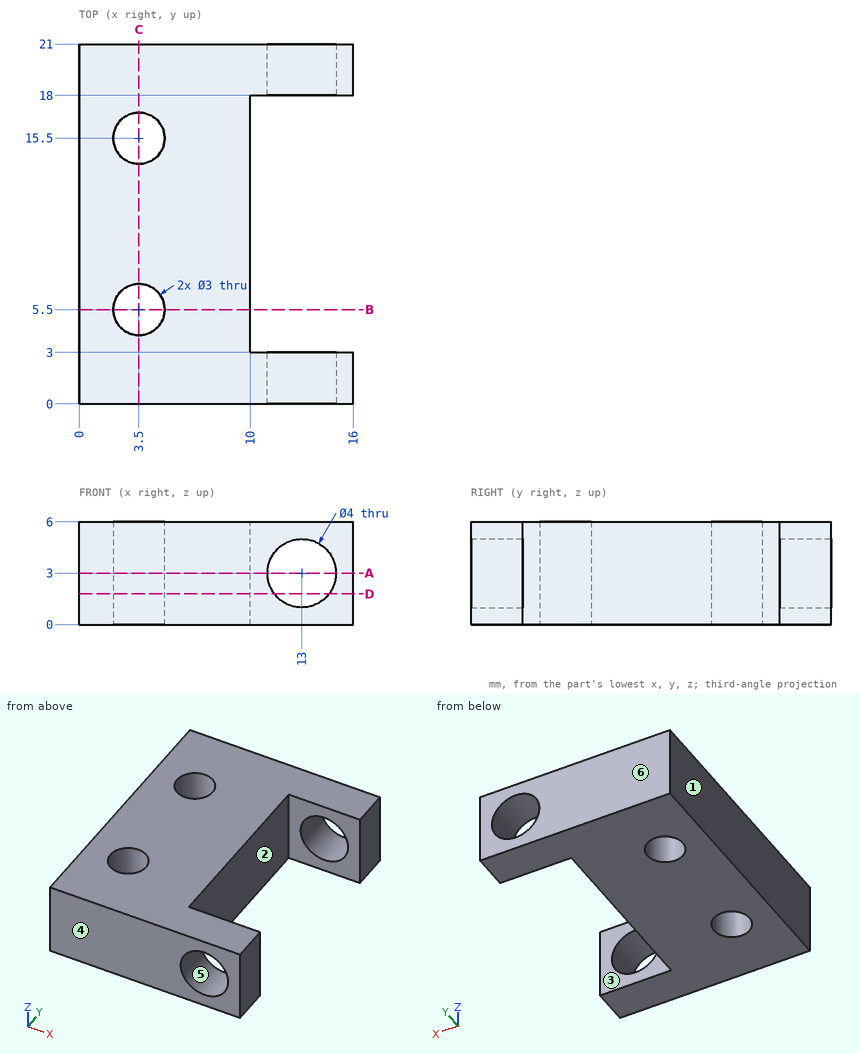
For this review, use the dimensioned drawing (mm, ordinates from the lowest corner) and the shaded views. A direction names the side the tool comes from. Round coordinates to 2 decimals unless told otherwise and drop trailing zeros. Write each loop counter-clockwise with the first axis right and the second up, starting at its lowest first coordinate (ties: lowest second). Pieces come first, ordered by that corner, then holes. Notation, with made-up numbers: M -39.5,-38.5 L 0.5,-38.5 A31 cw 0.5,-3.5 Z; hole C -33.5,4.5 d1. An arc over 180 degrees is marked long. Answer as CSV lines item,"result". Start each with the question number.
Q1. The part is to be moulded in two halves that separate along Y. For the marked faces 3, 4, 5 and 6, say which applies: +Y half, -Y half, draft (parallel to the pull), parting line (faces both ways), or undercut.
Q2. Clearance check with a flat-ended pin moving along its axis: P1, Ø1, axis at y = 12, z = 1, coming from the +X side. State where the tip first meets the part, or that it passes through.
Q3. Consider section D-D, the plane z = 1.8. Give the boundary of the cut face in (x, y), then the cut area to 3 significant figures.
Q4. Consider section A-A, the plane z = 3. Give the boundary of the cut face in (x, y).
Q5. Wall thickness on line 1 along Y through (x, z) = (3.5, 2.95); line 2 along X through (y, z) = (20.05, 3); line 3 along X through (y, z) = (15.5, 3.1): over which ranges is each line inside the solid? List them lowest first.
Q6. Consider section C-C, the plane x = 3.5. Give the boundary of the cut face in (y, z), then the cut area to 3 significant figures.
Q7. Consider section B-B, the plane y = 5.5. Give the boundary of the cut face in (x, z), then the cut area to 3 significant figures.
Q8. Tool access review of the marked faces 1 and 2: name each direction out of +Z, -Z, +X, -X, +Y, -Y from which nothing blocks a thin tool from reaching the whole face with its end or side.
Result set:
1,face 3,"undercut"
1,face 4,"-Y half"
1,face 5,"draft"
1,face 6,"+Y half"
2,P1,"stops at x = 10"
3,outline,"M 0,0 L 11.4,0 L 11.4,3 L 10,3 L 10,18 L 11.4,18 L 11.4,21 L 0,21 Z; M 14.6,0 L 16,0 L 16,3 L 14.6,3 Z; M 14.6,18 L 16,18 L 16,21 L 14.6,21 Z; hole C 3.5,5.5 d3; hole C 3.5,15.5 d3"
3,area,"213 mm²"
4,outline,"M 0,0 L 11,0 L 11,3 L 10,3 L 10,18 L 11,18 L 11,21 L 0,21 Z; M 15,0 L 16,0 L 16,3 L 15,3 Z; M 15,18 L 16,18 L 16,21 L 15,21 Z; hole C 3.5,5.5 d3; hole C 3.5,15.5 d3"
5,line 1,"y = 0 to 4, 7 to 14, 17 to 21"
5,line 2,"x = 0 to 11, 15 to 16"
5,line 3,"x = 0 to 2, 5 to 10"
6,outline,"M 0,0 L 4,0 L 4,6 L 0,6 Z; M 7,0 L 14,0 L 14,6 L 7,6 Z; M 17,0 L 21,0 L 21,6 L 17,6 Z"
6,area,"90.0 mm²"
7,outline,"M 0,0 L 2,0 L 2,6 L 0,6 Z; M 5,0 L 10,0 L 10,6 L 5,6 Z"
7,area,"42.0 mm²"
8,face 1,"+Z, -Z, -X, +Y, -Y"
8,face 2,"+Z, -Z, +X"
